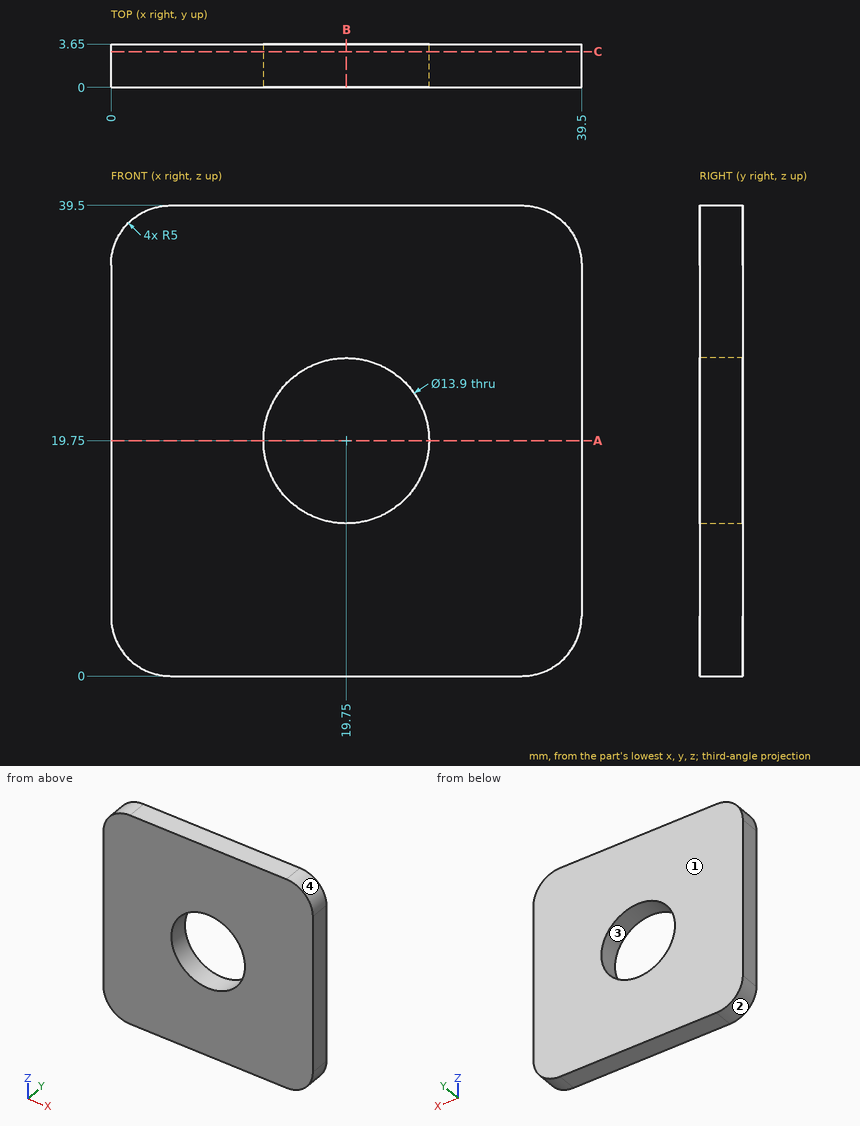
Verification items for this drawing (mm, ordinates from the low corner). Give positions to 0.01 mm unless a question says otherwise; leave off trailing zeros. Write each loop counter-clockwise with the first axis right and the second up, starting at its lowest first coordinate (ties: lowest second). Pieces come first, ordered by that corner, then holes. Notation, with made-up numbers: M 50.5,31 L 86.5,31 A12 ccw 86.5,53 Z; hole C 62,28 d2. An arc over 180 degrees is marked long. Use one line per item in the form item = value.
(1) Material ranges on line 1 along Z through (x, y) = (19.75, 2.45); line 2 along X through (y, z) = (2.15, 17.5), recorded low to high.
Answer block:
line_1 = 0 to 12.8, 26.7 to 39.5
line_2 = 0 to 13.17, 26.33 to 39.5
(2) Draft check along X on the marked faces 1, 2, 3 and 4. Enter one of: pulls with the +X half, pulls with the -X half, needs draft (parallel to the pull), parting line crosses it, or undercut.
Answer block:
face_1 = needs draft
face_2 = pulls with the -X half
face_3 = undercut
face_4 = pulls with the +X half
(3) Section check A-A on z = 19.75. Record the boundary of the cut face in (x, y), plus the area to 3 significant figures.
Answer block:
outline = M 0,0 L 12.8,0 L 12.8,3.65 L 0,3.65 Z; M 26.7,0 L 39.5,0 L 39.5,3.65 L 26.7,3.65 Z
area = 93.4 mm2
(4) Section check B-B on x = 19.75. Record the boundary of the cut face in (y, z).
Answer block:
outline = M 0,0 L 3.65,0 L 3.65,12.8 L 0,12.8 Z; M 0,26.7 L 3.65,26.7 L 3.65,39.5 L 0,39.5 Z
(5) Section check C-C on y = 3. Record the boundary of the cut face in (x, z), plus the area to 3 significant figures.
Answer block:
outline = M 0,5 A5 ccw 5,0 L 34.5,0 A5 ccw 39.5,5 L 39.5,34.5 A5 ccw 34.5,39.5 L 5,39.5 A5 ccw 0,34.5 Z; hole C 19.75,19.75 d13.9
area = 1,390 mm2
